from build123d import *

# Parameters (mm, degrees)
SKETCH2_W           = 100
SKETCH2_H           = 100
SKETCH2_R           = 3
BOSS_EXTRUDE1_DEPTH = 1.8
FILLET1_R           = 6
SKETCH3_R           = 42
SKETCH3_R_2         = 40
BOSS_EXTRUDE2_DEPTH = 3


with BuildPart() as part:
    # Sketch2 → Boss-Extrude1 (new body)
    with BuildSketch(Plane(origin=(0, 0, 0), x_dir=(1, 0, 0), z_dir=(0, 1, 0))):
        Rectangle(SKETCH2_W, SKETCH2_H)
        with Locations(Location((-42.425, 42.425, 0), (0, 0, 270))):
            Circle(SKETCH2_R, mode=Mode.SUBTRACT)
        with Locations(Location((42.425, 42.425, 0), (0, 0, 270))):
            Circle(SKETCH2_R, mode=Mode.SUBTRACT)
        with Locations(Location((42.425, -42.425, 0), (0, 0, 270))):
            Circle(SKETCH2_R, mode=Mode.SUBTRACT)
        with Locations(Location((-42.425, -42.425, 0), (0, 0, 270))):
            Circle(SKETCH2_R, mode=Mode.SUBTRACT)
    extrude(amount=BOSS_EXTRUDE1_DEPTH)

    # Fillet1
    fillet1_edges = [part.edges().sort_by_distance(p)[0] for p in [
        (50, 0.9, 50),
        (-50, 0.9, 50),
        (-50, 0.9, -50),
        (50, 0.9, -50),
    ]]
    fillet(fillet1_edges, radius=FILLET1_R)

    # Sketch3 → Boss-Extrude2 (add)
    with BuildSketch(Plane.XZ):
        with Locations(Location((0, 0, 0), (0, 0, 90))):
            Circle(SKETCH3_R)
        with Locations(Location((0, 0, 0), (0, 0, 270))):
            Circle(SKETCH3_R_2, mode=Mode.SUBTRACT)
    extrude(amount=BOSS_EXTRUDE2_DEPTH)


solid = part.part
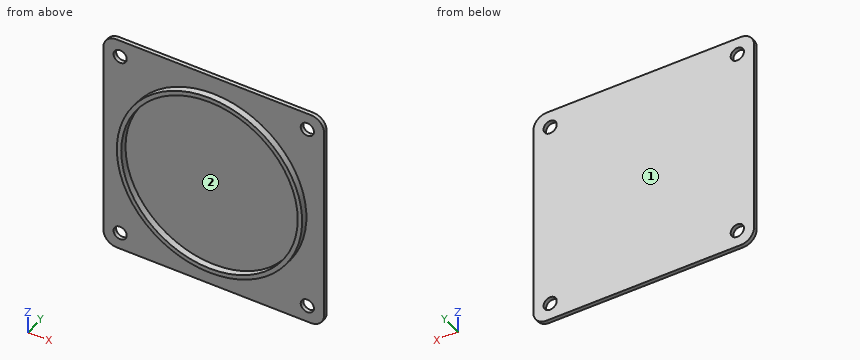
CAD build for the part. Positions are in the model's coordinates, mm. Face numbers are marked on the shaded views. Round coordinates to 2 decimals unless told otherwise and drop trailing zeros. Order: outer loops, then holes, each group sorted by start corner. A loop starts at its lowest first (then second) coordinate and runs counter-clockwise, first axis right, second up. Notation, with made-up numbers: M 16.25,86.25 L 28.25,86.25 A25 cw 28.25,100.25 Z; hole C 4,75.25 d7. An arc over 180 degrees is marked long. Use one line per item in the form item = value.
Q1. Saw through at A-A on x = 0. Give the cut face in (y, z), then the cut area to 3 significant figures.
Recorded:
outline = M -3,-42 L 0,-42 L 0,-50 L 1.8,-50 L 1.8,50 L 0,50 L 0,42 L -3,42 L -3,40 L 0,40 L 0,-40 L -3,-40 Z
area = 192 mm^2
Q2. Saw through at B-B on z = -9.5. Give the cut face in (x, y), then the cut area to 3 significant figures.
Recorded:
outline = M -50,0 L -40.91,0 L -40.91,-3 L -38.86,-3 L -38.86,0 L 38.86,0 L 38.86,-3 L 40.91,-3 L 40.91,0 L 50,0 L 50,1.8 L -50,1.8 Z
area = 192 mm^2
Q3. Two-plate mould, pull along Z, no slides. Class the marked faces 1 and 2: +Z half, -Z half, draft (parallel to the pull), parting line (faces both ways), or undercut.
Recorded:
face_1 = draft
face_2 = undercut
Q4. Flat gauge pin, fed straight in: P1, Ø6, axis at x = 14, z = 20.5, coming from the -Y side. Where does the tip first touch, or does it go through?
Recorded:
P1 = 0
Q5. Saw through at C-C on y = -1.6. Give the cut face in (x, z).
Recorded:
outline = C 0,0 d84; hole C 0,0 d80
Q6. Probe L1, parallel to Z at x = -43, y = 1; L2, parallel to Y at x = 2, z = 23.5; L3, parallel to X at y = -2.25, z = 0. List the from-to ranges inside material, lowest first.
Recorded:
L1 = -50 to -45.37, -39.48 to 39.48, 45.37 to 50
L2 = 0 to 1.8
L3 = -42 to -40, 40 to 42
